The figure shows three views and two pictorial views of one solid part (mm, origin at its lowest corner). Answer the questions. Give positions to 0.01 mm unless a question says otherwise; leave off trailing zeros. Loops run counter-clockwise (first coordinate to the right, second up) from the corner with the lowest first, then second, coordinate; pieces in that order, holes last.
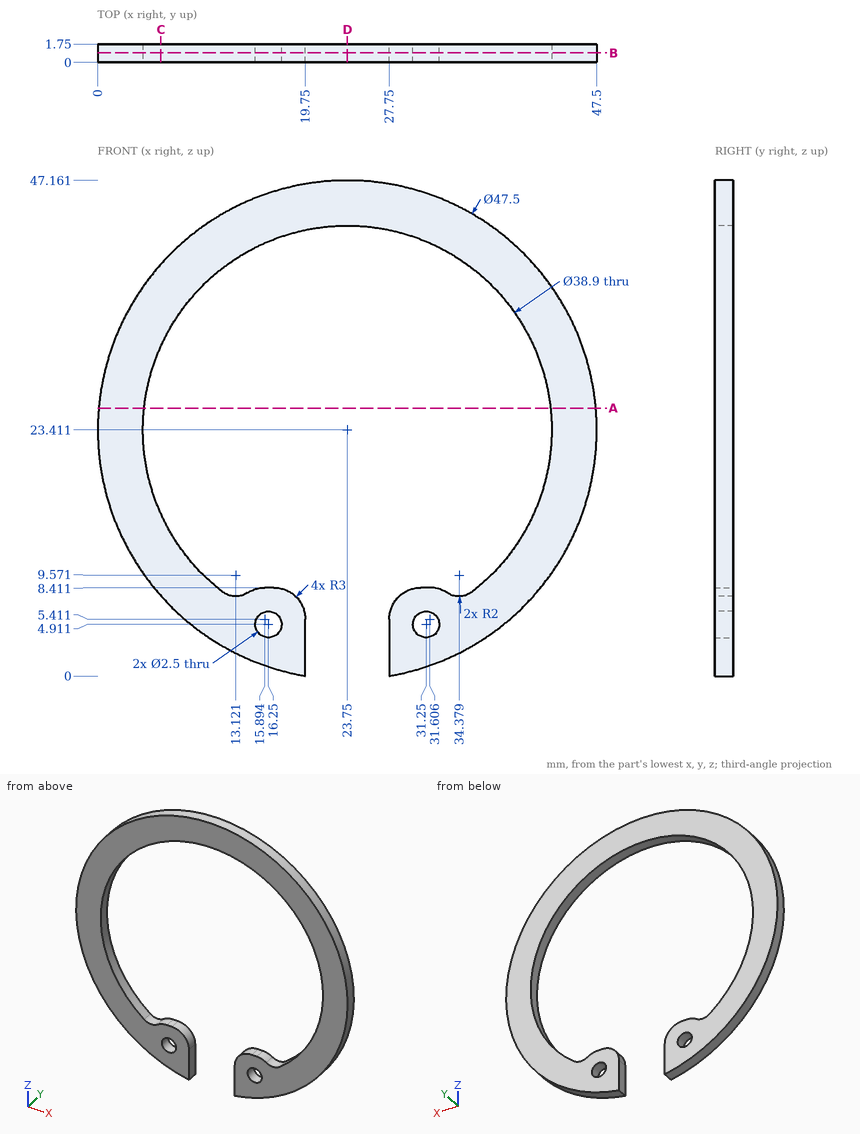
Q1. Section A-A on z = 25.5 is taken. Give the vertices of the cut face in (x, y).
Q2. Given pin 1 (0.9 mm diameter, centred on x = 16, y = 0.5, fed in from +Z); pin 2 (0.5 mm diameter, centred on y = 1.5, z = 4, fed in from +X), each flat-ended and moving along its own axis, determine where each tip first touches the part or whether it passes through.
Q3. Section B-B on y = 0.9 is taken. State how many separate pieces and enclosed holes the cut face has, plus the area to 3 significant figures.
Q4. Section D-D on x = 23.75 is taken. Give the vertices of the cut face in (y, z).
Q5. Section C-C on x = 6 is taken. Give the vertices of the cut face in (y, z), plus the area to 3 significant figures.
Q6. Consider line 1 along X through (y, z) = (0.5, 8) (1 decimal); line 2 along Z through (x, y) = (23.75, 1.25); line 3 along X through (y, z) = (0.1, 40.5) (1 decimal). Determine where each line is inside the solid, lowest interval first.
Check result:
1. outline: (0.09, 0) - (4.41, 0) - (4.41, 1.75) - (0.09, 1.75) - close; (43.09, 0) - (47.41, 0) - (47.41, 1.75) - (43.09, 1.75) - close
2. pin 1: stops at z = 46.01
2. pin 2: stops at x = 37.78
3. separate pieces: 1
3. enclosed holes: 2
3. area: 572 mm2
4. outline: (0, 42.86) - (1.75, 42.86) - (1.75, 47.16) - (0, 47.16) - close
5. outline: (0, 7.63) - (1.75, 7.63) - (1.75, 15.46) - (0, 15.46) - close; (0, 31.36) - (1.75, 31.36) - (1.75, 39.19) - (0, 39.19) - close
5. area: 27.4 mm2
6. line 1: x = 5.7 to 11.9, 14.4 to 18.3, 29.2 to 33.1, 35.6 to 41.8
6. line 2: z = 42.86 to 47.16
6. line 3: x = 7.3 to 14.5, 33 to 40.2
